from build123d import *

# Parameters (mm, degrees)
F1_DEPTH  = 1.54
F3_D      = 3.3
F5_DEPTH  = 25
F8_DEPTH  = 10
F10_DEPTH = 7.5


# Not quite as in the source:
# - a pattern or mirror of a feature is missing from the dataset's text; its kind, count and spacing are read off the source's solid


with BuildPart() as f1:
    # F0 (on Top) → F1 (new body)
    with BuildSketch(Plane.XY):
        with BuildLine():
            Line((-19.5, -27.75), (19.5, -27.75))
            ThreePointArc((19.5, -27.75), (23.7426406871, -25.9926406871), (25.5, -21.75))
            Line((25.5, -21.75), (25.5, 21.75))
            ThreePointArc((25.5, 21.75), (23.7426406871, 25.9926406871), (19.5, 27.75))
            Line((19.5, 27.75), (-19.5, 27.75))
            ThreePointArc((-19.5, 27.75), (-23.7426406871, 25.9926406871), (-25.5, 21.75))
            Line((-25.5, 21.75), (-25.5, -21.75))
            ThreePointArc((-25.5, -21.75), (-23.7426406871, -25.9926406871), (-19.5, -27.75))
        make_face()
    extrude(amount=F1_DEPTH)

    # F3 (through all)
    with Locations(Plane.XY.offset(1.54)):
        with Locations((-19.45, 22.8), (19.45, 22.8), (-19.45, -22.8), (19.45, -22.8)):
            Hole(F3_D / 2)

    # F4 (on face) → F5 (join)
    with BuildSketch(Plane.XY.offset(1.54)):
        Polygon((10.85, 9.65), (11.5, 9.65), (11.5, 25.65), (10.85, 25.65), (10.85, 13.7976789847), (7.03, 13.7976789847), (7.03, 25.65), (6.38, 25.65), (6.38, 13.7976789847), (2.56, 13.7976789847), (2.56, 25.65), (1.91, 25.65), (1.91, 13.7976789847), (-1.91, 13.7976789847), (-1.91, 25.65), (-2.56, 25.65), (-2.56, 13.7976789847), (-6.38, 13.7976789847), (-6.38, 25.65), (-7.03, 25.65), (-7.03, 13.7976789847), (-10.85, 13.7976789847), (-10.85, 25.65), (-11.5, 25.65), (-11.5, 9.65), (-10.85, 9.65), (-10.85, 13.1476789847), (10.85, 13.1476789847), align=None)
    extrude(amount=F5_DEPTH)

    # F7 (on offset) → F8 (join)
    with BuildSketch(Plane.XZ.offset(7.75)):
        Polygon((18.1, 1.54), (25.5, 1.54), (25.5, 8.04), (24.5, 11.54), (20.1, 11.54), (18.1, 8.04), align=None)
    f8 = extrude(amount=-F8_DEPTH)

    # F8_copies: F8 across plane
    add(f8.mirror(Plane(origin=(0, 0, 0), x_dir=(0, 0, -1), z_dir=(-1, 0, 0))))

    # F9 (on Right) → F10 (join, symmetric)
    with BuildSketch(Plane.YZ):
        Polygon((-27.75, 1.54), (-20.35, 1.54), (-20.35, 8.04), (-22.35, 11.54), (-26.75, 11.54), (-27.75, 8.04), align=None)
    extrude(amount=F10_DEPTH, both=True)


solid = f1.part
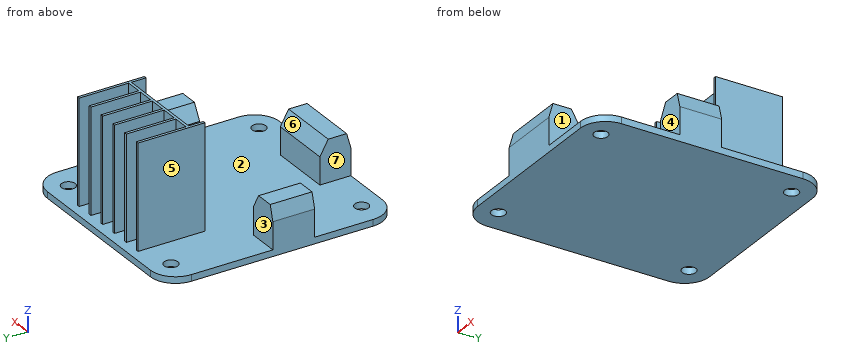
Read the model definition and answer for the solid it produces. Units are mm, in the model's axes. Face numbers are marked on the shaded views. A direction names the side the tool comes from. Coordinates: 2 decimals unless noted, no trailing zeros. Write each loop counter-clockwise with the first axis right and the second up, starting at its lowest first coordinate (ties: lowest second). Pieces come first, ordered by that corner, then holes. Notation, with made-up numbers: (3, 63) - (52, 63) arc R26 ccw to (52, 96) - close; hole circle Ø5 at (-16, -29). An arc over 180 degrees is marked (long way). One line per question, with ' | ' between items.
Q1. Consider L1, parallel to Y at x = -19.45, z = 1.15; L2, parallel to X at y = 20, z = 14.75; L3, parallel to X at y = -7.5, z = 2.25. Determine where each line is inside the solid, lowest interval first. Write a range as [from, to].
Result set:
L1: [-27.75, -24.45], [-21.15, 21.15], [24.45, 27.75] | L2: [-11.5, -10.85], [-7.03, -6.38], [-2.56, -1.91], [1.91, 2.56], [6.38, 7.03], [10.85, 11.5] | L3: [-25.5, -18.1], [18.1, 25.5]
Q2. Determine the mould class of the marked faces 1, 2 and 3 for opening direction X: +X half, -X half, draft (parallel to the pull), parting line (faces both ways), or undercut.
Result set:
face 1: +X half | face 2: undercut | face 3: draft
Q3. For the marked faces 4, 5, 6 and 7, determine the directions among +Z, -Z, +X, -X, +Y, -Y from which every point of the face is accessible in a straight line to the end or side of a thin tool.
Result set:
face 4: +Z, +X, -X, -Y | face 5: +Z, -X, +Y, -Y | face 6: +Z, +X, -X | face 7: +Z, -X, -Y
Q4. Find section A-A, the plane y = -5. Write down the section's boundary in (x, z).
Result set:
outline: (-25.5, 0) - (25.5, 0) - (25.5, 8.04) - (24.5, 11.54) - (20.1, 11.54) - (18.1, 8.04) - (18.1, 1.54) - (-18.1, 1.54) - (-18.1, 8.04) - (-20.1, 11.54) - (-24.5, 11.54) - (-25.5, 8.04) - close
Q5. Find section B-B, the plane z = 13. Write down the section's boundary in (x, y).
Result set:
outline: (-11.5, 9.65) - (-10.85, 9.65) - (-10.85, 13.15) - (10.85, 13.15) - (10.85, 9.65) - (11.5, 9.65) - (11.5, 25.65) - (10.85, 25.65) - (10.85, 13.8) - (7.03, 13.8) - (7.03, 25.65) - (6.38, 25.65) - (6.38, 13.8) - (2.56, 13.8) - (2.56, 25.65) - (1.91, 25.65) - (1.91, 13.8) - (-1.91, 13.8) - (-1.91, 25.65) - (-2.56, 25.65) - (-2.56, 13.8) - (-6.38, 13.8) - (-6.38, 25.65) - (-7.03, 25.65) - (-7.03, 13.8) - (-10.85, 13.8) - (-10.85, 25.65) - (-11.5, 25.65) - close
Q6. Find section D-D, the plane y = 17. Write down the section's boundary in (x, z), plus the area to 3 significant figures.
Result set:
outline: (-25.5, 0) - (25.5, 0) - (25.5, 1.54) - (11.5, 1.54) - (11.5, 26.54) - (10.85, 26.54) - (10.85, 1.54) - (7.03, 1.54) - (7.03, 26.54) - (6.38, 26.54) - (6.38, 1.54) - (2.56, 1.54) - (2.56, 26.54) - (1.91, 26.54) - (1.91, 1.54) - (-1.91, 1.54) - (-1.91, 26.54) - (-2.56, 26.54) - (-2.56, 1.54) - (-6.38, 1.54) - (-6.38, 26.54) - (-7.03, 26.54) - (-7.03, 1.54) - (-10.85, 1.54) - (-10.85, 26.54) - (-11.5, 26.54) - (-11.5, 1.54) - (-25.5, 1.54) - close | area: 176 mm^2
Q7. Each of these flat-tipped pins is pushed along its axis until it touches: P1, Ø4.5, axis at x = 19.45, y = 22.8, coming from the +Z side; P2, Ø8, axis at x = -5.5, z = 13.5, coming from the +Y side; P3, Ø6, axis at y = 18, z = 8, coming from the -X side; P4, Ø2, axis at x = -19.45, y = -22.8, coming from the -Z side. Where does it stop, or does it pass through?
Result set:
P1: z = 1.54 | P2: y = 25.65 | P3: x = -11.5 | P4: through
Q8. Find section C-C, the plane z = 2.75. State how many separate pieces and enclosed holes the cut face has, plus the area to 3 significant figures.
Result set:
separate pieces: 4 | enclosed holes: 0 | area: 325 mm^2
